Could you check a few things on this model? Use its own coordinates, in mm. A direction names the side the tool comes from. Give positions to 0.01 mm unless a question says otherwise; leave off trailing zeros. Loops run counter-clockwise (first coordinate to the right, second up) from the corner with the lowest first, then second, coordinate; pieces in that order, holes last. Notation, with made-up numbers: (83, 50) -> (116, 50) arc R11 ccw to (116, 71) -> close; hole circle Ø4 at (40.5, -3). An arc over 180 degrees is marked (long way). Write item = value, one per line. Start each with the question number.
1) I'm going to push flat-ended pins straight in: pin 1 Ø3 at (x, y) = (-18, 2) entering from -Z; pin 2 Ø2.5 at (x, y) = (1.5, -1) entering from +Z; pin 3 Ø1 at (y, z) = (1, 9.5) entering from -X. Where does each tip first touch, or does it pass through?
2) I need wall thicknesses on probe 1 along Z at (x, y) = (27, -0.75); probe 2 along Z at (x, y) = (-22, 1.4); probe 3 along Z at (x, y) = (28, -0.25). Which ranges of each line are inside material? Lowest first, please. Write a range as from..to.
3) I want a section at A-A (z = 0). List the corners of the cut face in (x, y) for me, and give its area (3 significant figures).
4) I want a section at D-D (z = -47). List the corners of the cut face in (x, y) for me, and give its area (3 significant figures).
5) I want a section at B-B (x = 0). List the corners of the cut face in (y, z) for me.
6) I want a section at C-C (y = -0.7). List the corners of the cut face in (x, z) for me (1 decimal), and give its area (3 significant figures).
7) If we mould it in two halves opening along Z, with no side actions, what happens to faces 4 (the face through (-28.19, 0.04, 16.37)), 5 (the face through (-52.716, 0.035, -11.706)), 6 (the face through (-32, 2.5, 16))? For each: +Z half, -Z half, draft (parallel to the pull), parting line (faces both ways), or undercut.
8) On a 3-axis mill with a long thin cutter (end or side, diameter ignored), from which of +Z, -Z, +X, -X, +Y, -Y can I reach the whole of each face in a straight line? I mean faces 1 (the face through (32.25, 1.49, 12.98)), 2 (the face through (1, -2.5, -37)), 3 (the face through (26.827, -0.979, 22.273)). Say none if no direction works.
from build123d import *

# Parameters (mm, degrees)
SKETCH1_R                = 54
SKETCH1_R_2              = 37.6
BOSS_EXTRUDE1_DEPTH      = 2.5
BOSS_EXTRUDE2_DEPTH      = 2.5
FILLET1_R                = 0.8
CIRPATTERN1_COUNT        = 3
FILLET1_OF_CIRPATTERN1_R = 0.8
CHAMFER2_SIZE            = 2


with BuildPart() as part:
    # Sketch1 → Boss-Extrude1 (new, symmetric)
    with BuildSketch(Plane(origin=(0, 0, 0), x_dir=(1, 0, 0), z_dir=(0, 1, 0))):
        with Locations(Location((0, 0, 0), (0, 0, 270))):
            Circle(SKETCH1_R)
        with Locations(Location((0, 0, 0), (0, 0, 270))):
            Circle(SKETCH1_R_2, mode=Mode.SUBTRACT)
    extrude(amount=BOSS_EXTRUDE1_DEPTH, both=True)

    # Sketch2 → Boss-Extrude2 (add, symmetric)
    with BuildSketch(Plane(origin=(0, 0, 0), x_dir=(1, 0, 0), z_dir=(0, 1, 0))):
        with BuildLine():
            Line((-5.875, 32.6), (5.875, 32.6))
            Line((5.875, 32.6), (5.875, 37.138179479))
            ThreePointArc((5.875, 37.138179479), (0, 37.6), (-5.875, 37.138179479))
            Line((-5.875, 37.138179479), (-5.875, 32.6))
        make_face()
    boss_extrude2 = extrude(amount=BOSS_EXTRUDE2_DEPTH, both=True)

    # Fillet1
    fillet1_edges = [part.edges().sort_by_distance(p)[0] for p in [
        (-5.875, 0, -37.138179479),
        (5.875, 0, -37.138179479),
    ]]
    fillet(fillet1_edges, radius=FILLET1_R)

    # CirPattern1: Boss-Extrude2 ×3 about axis
    cirpattern1_axis = Axis((0, 0, 0), (0, 1, 0))
    for i in range(1, CIRPATTERN1_COUNT):
        add(boss_extrude2.rotate(cirpattern1_axis, i * 360 / CIRPATTERN1_COUNT))

    # Fillet1 of CirPattern1
    fillet1_of_cirpattern1_edges = [part.edges().sort_by_distance(p)[0] for p in [
        (-29.225106879, 0, 23.656988987),
        (-35.100106879, 0, 13.481190492),
        (35.100106879, 0, 13.481190492),
        (29.225106879, 0, 23.656988987),
    ]]
    fillet(fillet1_of_cirpattern1_edges, radius=FILLET1_OF_CIRPATTERN1_R)

    # Chamfer2
    chamfer2_edges = [part.edges().sort_by_distance(p)[0] for p in [
        (5.875, 2.5, -34.394780843),
        (-32.562555182, 2.5, -18.8),
        (-5.875, 2.5, -34.394780843),
        (6.163183117, 2.5, -36.804414089),
        (-6.163183117, 2.5, -36.804414089),
        (26.849253967, 2.5, 22.285289669),
        (-32.724253967, 2.5, 12.109491174),
        (32.724253967, 2.5, 12.109491174),
        (32.562555182, 2.5, -18.8),
        (28.791966014, 2.5, 23.739680192),
        (34.955149131, 2.5, 13.064733897),
        (-26.849253967, 2.5, 22.285289669),
        (0, 2.5, 37.6),
        (-34.955149131, 2.5, 13.064733897),
        (-28.791966014, 2.5, 23.739680192),
    ]]
    chamfer(chamfer2_edges, length=CHAMFER2_SIZE)


solid = part.part
Answer list:
q1.pin_1 = -51.42
q1.pin_2 = 54
q1.pin_3 = -53.24
q2.probe_1 = -46.77..-26.17, 18.43..22.37, 26.17..46.77
q2.probe_2 = -49.32..-31.6, 31.6..49.32
q2.probe_3 = -46.17..-25.1, 16.7..22.95, 25.1..46.17
q3.outline = (-54, -2.5) -> (-37.6, -2.5) -> (-37.6, 0.5) -> (-39.6, 2.5) -> (-54, 2.5) -> close; (37.6, -2.5) -> (54, -2.5) -> (54, 2.5) -> (39.6, 2.5) -> (37.6, 0.5) -> close
q3.area = 160 mm^2
q4.outline = (-26.59, -2.5) -> (26.59, -2.5) -> (26.59, 2.5) -> (-26.59, 2.5) -> close
q4.area = 266 mm^2
q5.outline = (-2.5, -54) -> (2.5, -54) -> (2.5, -32.6) -> (-2.5, -32.6) -> close; (-2.5, 37.6) -> (0.5, 37.6) -> (2.5, 39.6) -> (2.5, 54) -> (-2.5, 54) -> close
q6.outline = circle Ø108 at (0, 0); hole (-35.4, 12.6) arc R37.6 ccw to (-6.8, -37) arc R0.8 ccw to (-5.9, -36.2) -> (-5.9, -32.6) -> (5.9, -32.6) -> (5.9, -36.2) arc R0.8 ccw to (6.8, -37) arc R37.6 ccw to (35.4, 12.6) arc R0.8 ccw to (34.3, 13) -> (31.2, 11.2) -> (25.3, 21.4) -> (28.4, 23.2) arc R0.8 ccw to (28.6, 24.4) arc R37.6 ccw to (-28.6, 24.4) arc R0.8 ccw to (-28.4, 23.2) -> (-25.3, 21.4) -> (-31.2, 11.2) -> (-34.3, 13) arc R0.8 ccw to start
q6.area = 4,890 mm^2
q7.face_4 = undercut
q7.face_5 = parting line
q7.face_6 = draft
q8.face_1 = +Y
q8.face_2 = +Z, -Z, +X, -X, -Y
q8.face_3 = +Y, -Y
